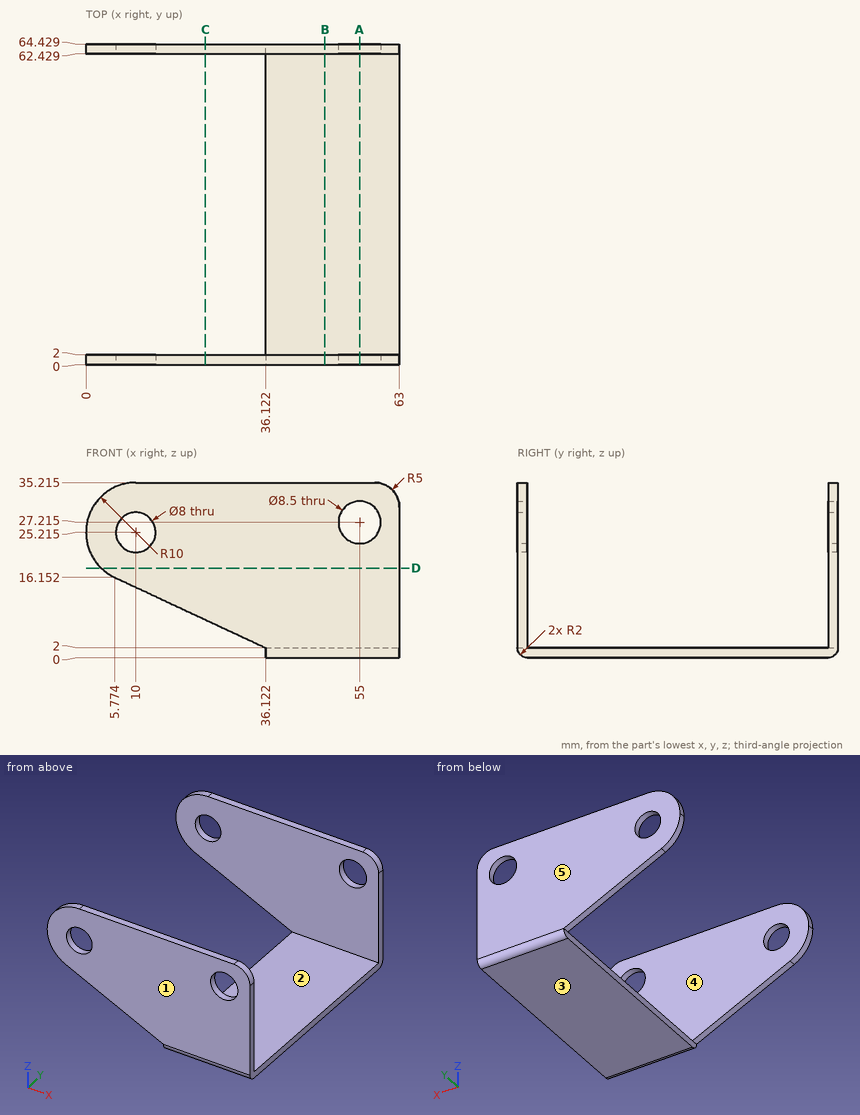
Verification items for this drawing (mm, ordinates from the low corner). A direction names the side the tool comes from. Coordinates: 2 decimals unless noted, no trailing zeros. Loops run counter-clockwise (first coordinate to the right, second up) from the corner with the lowest first, then second, coordinate; pieces in that order, holes last. Notation, with made-up numbers: (81, 28) - (138, 28) arc R18 ccw to (138, 45) - close; hole circle Ø11 at (80, -34). An arc over 180 degrees is marked (long way). One line per item, written item: value. Start each with the question number.
(1) Cross-section at A-A on x = 55. Enter the section's corners in (y, z) (1 decimal).
(2) Cross-section at C-C on x = 24. Enter the section's corners in (y, z) (1 decimal).
(3) Cross-section at B-B on x = 48. Enter the section's corners in (y, z) (1 decimal).
(4) Mould release check, pull along Y, two halves, no side actions. Record for the marked faces 1, 2 and 3: released by +Y, released by -Y, zero draft, split by the parting line, or undercut.
(5) Material ranges on line 1 (Y direction, x = 16, z = 33.5); line 2 (Z direction, x = 10, y = 63) (1 decimal); line 3 (Z direction, x = 44, y = 22), recorded low to high. Write a range as [from, to].
(6) Cross-section at D-D on z = 18. Enter the section's corners in (x, y) (1 decimal).
(7) Depth check by flat-ended pin: P1, Ø21.5, axis at x = 48.5, y = 18.5, coming from the +Z side; P2, Ø5, axis at x = 10, z = 25.21, coming from the +Y side; P3, Ø10, axis at x = 24, y = 58, coming from the -Z side; P4, Ø2, axis at y = 33, z = 1, coming from the -X side. Enter the tip coordinate at first touch or a pass-through.
(8) Tool access check on the marked faces 4 and 5. Record the directions out of +Z, -Z, +X, -X, +Y, -Y that give a thin tool (end or side, any length) a straight path to the whole face; none if there is none.
Results below:
1. outline: (0, 2) arc R2 ccw to (2, 0) - (62.4, 0) arc R2 ccw to (64.4, 2) - (64.4, 23) - (62.4, 23) - (62.4, 2) - (2, 2) - (2, 23) - (0, 23) - close; (0, 31.5) - (2, 31.5) - (2, 35.2) - (0, 35.2) - close; (62.4, 31.5) - (64.4, 31.5) - (64.4, 35.2) - (62.4, 35.2) - close
2. outline: (0, 7.7) - (2, 7.7) - (2, 35.2) - (0, 35.2) - close; (62.4, 7.7) - (64.4, 7.7) - (64.4, 35.2) - (62.4, 35.2) - close
3. outline: (0, 2) arc R2 ccw to (2, 0) - (62.4, 0) arc R2 ccw to (64.4, 2) - (64.4, 35.2) - (62.4, 35.2) - (62.4, 2) - (2, 2) - (2, 35.2) - (0, 35.2) - close
4. face 1: released by -Y
4. face 2: undercut
4. face 3: zero draft
5. line 1: y = [0, 2], [62.43, 64.43]
5. line 2: z = [14.2, 21.2], [29.2, 35.2]
5. line 3: z = [0, 2]
6. outline: (3.1, 0) - (63, 0) - (63, 2) - (3.1, 2) - close; (3.1, 62.4) - (63, 62.4) - (63, 64.4) - (3.1, 64.4) - close
7. P1: stops at z = 2
7. P2: passes through
7. P3: stops at z = 6.57
7. P4: stops at x = 36.12
8. face 4: +Z, +X, -X
8. face 5: +Z, -Z, +X, -X, +Y
